Solid Edge part; units mm, degrees
sketch "Sketch1" plane through (0, 0, 0) normal (0, 0, 1) x (1, 0, 0)
  line L0 (0, -121.1263) -> (205, -121.1263)
  line L1 (205, -121.1263) -> (205, 23.8737)
  line L2 (205, 23.8737) -> (0, 23.8737)
  line L3 (0, 23.8737) -> (0, -121.1263)
extrude "Protrusion1" add sketch "Sketch1" along normal blind 10
hole "Hole1" at (198.5, -61.1263, 10) direction (0, 0, -1) diameter 8.3 end through all
hole "Hole2" at (198.5, -101.1263, 10) direction (0, 0, -1) diameter 8.3 end through all
hole "Hole3" at (6.5, -101.1263, 10) direction (0, 0, -1) diameter 8.3 end through all
hole "Hole4" at (6.5, -61.1263, 10) direction (0, 0, -1) diameter 8.3 end through all
hole "Hole_7" at (34.5, -8.6263, 0) direction (0, 0, 1) diameter 17.5 depth 50.8 countersink diameter 31 countersink angle 90
hole "Hole5" at (34.5, -81.6263, 0) direction (0, 0, 1) diameter 17.5 depth 50.8 countersink diameter 31 countersink angle 90
hole "Hole6" at (170.5, -81.6263, 0) direction (0, 0, 1) diameter 17.5 depth 50.8 countersink diameter 31 countersink angle 90
hole "Hole7" at (170.5, -8.6263, 0) direction (0, 0, 1) diameter 17.5 depth 50.8 countersink diameter 31 countersink angle 90
properties material "Aluminum, 6061-T6"
Check sheet for the modelled part. Datum: model origin and axes. Units: mm. Round coordinates to 2 decimals unless told otherwise and drop trailing zeros. Order: outer loops, then holes, each group sorted by start corner. A loop starts at its lowest first (then second) coordinate and runs counter-clockwise, first axis right, second up. Notation, with made-up numbers: M 9.25,-13.75 L 48.25,-13.75 A17 cw 48.25,7.25 Z; hole C -26.5,36 d6. An arc over 180 degrees is marked long. One line per item, written item: value. Start each with the question number.
1. Section check B-B on x = 170.5. Enter the section's corners in (y, z).
2. Section check C-C on z = 4.75. Give the number of separate pieces and of enclosed holes in the cut face, and give its area (3 significant figures).
3. Section check A-A on x = 6.5. Enter the section's corners in (y, z), and give its area (3 significant figures).
4. Scan lines: line 1 along Y through (x, z) = (34.5, 8.5); line 2 along Y through (x, z) = (198.5, 7); line 3 along X through (y, z) = (-77.5, 8.5). Record each from-to range of solid material in increasing order.
5. Release check for a two-part mould opening along X. For faces 1 (the flat face through (101, -48, 10)), 2 (the conical face through (34.9, -90.79, 6.33)), 3 (the flat face through (0, -48, 5)), 4 (the cylindrical face through (6.68, -56.98, 5.07)) record: released by +X, released by -X, zero draft, split by the parting line, or undercut.
6. Gauge pin test, flat ends, axial feed: P1, Ø11, axis at x = 6.5, y = -101.13, coming from the -Z side; P2, Ø20, axis at x = 34.5, y = -81.63, coming from the -Z side. Record the tip position at first contact, or that the pin passes through.
Results found:
1. outline: M -121.13,0 L -97.13,0 L -90.38,6.75 L -90.38,10 L -121.13,10 Z; M -72.88,6.75 L -66.13,0 L -24.13,0 L -17.38,6.75 L -17.38,10 L -72.88,10 Z; M 0.12,6.75 L 6.87,0 L 23.87,0 L 23.87,10 L 0.12,10 Z
2. separate pieces: 1
2. enclosed holes: 8
2. area: 28,100 mm^2
3. outline: M -121.13,0 L -105.28,0 L -105.28,10 L -121.13,10 Z; M -96.98,0 L -65.28,0 L -65.28,10 L -96.98,10 Z; M -56.98,0 L 23.87,0 L 23.87,10 L -56.98,10 Z
3. area: 1,280 mm^2
4. line 1: -121.13 to -90.38, -72.88 to -17.38, 0.12 to 23.87
4. line 2: -121.13 to -105.28, -96.98 to -65.28, -56.98 to 23.87
4. line 3: 0 to 26.78, 42.22 to 162.78, 178.22 to 205
5. face 1: zero draft
5. face 2: undercut
5. face 3: released by -X
5. face 4: undercut
6. P1: z = 0
6. P2: z = 5.5
